Model file for the job. Use its own axes, mm. A direction names the side the tool comes from. Coordinates: 2 decimals unless noted, no trailing zeros. Loops run counter-clockwise (first coordinate to the right, second up) from the corner with the lowest first, then second, coordinate; pieces in that order, holes last.
from build123d import *

# Parameters (mm, degrees)
BASE_FLANGE1_DEPTH         = 3.175
M3_5_CLEARANCE_HOLE1_D     = 3.75
F_5_2_5_2_DIAMETER_HOLE1_D = 5.2
F_3_2_3_2_DIAMETER_HOLE1_D = 3.2
M20_CLEARANCE_HOLE1_D      = 22.86


# Sheet-metal steps are written as plain solids
with BuildPart() as part:
    # Sketch11 → Base-Flange1 (new body)
    with BuildSketch(Plane.XY.offset(3.175)):
        with BuildLine():
            Line((-42, 51), (-42, 19))
            ThreePointArc((-42, 19), (-40.535533906, 15.464466094), (-37, 14))
            Line((-37, 14), (-5, 14))
            ThreePointArc((-5, 14), (-1.464466094, 12.535533906), (0, 9))
            Line((0, 9), (0, 5))
            ThreePointArc((0, 5), (1.464466094, 1.464466094), (5, 0))
            Line((5, 0), (15, 0))
            ThreePointArc((15, 0), (18.535533906, 1.464466094), (20, 5))
            Line((20, 5), (20, 35.499999523))
            Line((20, 35.499999523), (48, 35.499999523))
            ThreePointArc((48, 35.499999523), (51.535533906, 36.964465617), (53, 40.499999523))
            Line((53, 40.499999523), (53, 50))
            ThreePointArc((53, 50), (51.535533906, 53.535533906), (48, 55))
            Line((48, 55), (20, 55))
            Line((20, 55), (20, 75))
            ThreePointArc((20, 75), (18.535533906, 78.535533906), (15, 80))
            Line((15, 80), (5, 80))
            ThreePointArc((5, 80), (1.464466094, 78.535533906), (0, 75))
            Line((0, 75), (0, 61))
            ThreePointArc((0, 61), (-1.464466094, 57.464466094), (-5, 56))
            Line((-5, 56), (-37, 56))
            ThreePointArc((-37, 56), (-40.535533906, 54.535533906), (-42, 51))
        make_face()
    extrude(amount=-BASE_FLANGE1_DEPTH)

    # M3.5 Clearance Hole1 (through all)
    with Locations(Plane.XY.offset(3.175)):
        with Locations((17, 75), (3, 5), (3, 75), (17, 5)):
            Hole(M3_5_CLEARANCE_HOLE1_D / 2)

    # Ø5.2 (5.2) Diameter Hole1 (through all)
    with Locations(Plane.XY.offset(3.175)):
        with Locations((47.5, 45), (27.5, 45)):
            Hole(F_5_2_5_2_DIAMETER_HOLE1_D / 2)

    # Ø3.2 (3.2) Diameter Hole1 (through all)
    with Locations(Plane.XY.offset(3.175)):
        with Locations((-36.490941809, 50.490941809), (-5.509058191, 50.490941809), (-5.509058191, 19.509058191), (-36.490941809, 19.509058191)):
            Hole(F_3_2_3_2_DIAMETER_HOLE1_D / 2)

    # M20 Clearance Hole1 (through all)
    with Locations(Plane.XY.offset(3.175)):
        with Locations((-21, 35)):
            Hole(M20_CLEARANCE_HOLE1_D / 2)


solid = part.part
Q1. Mould opens along Y. For faces 3 (the flat face through (20, 20, 2)), 4 (the flat face through (10, 80, 2)), 5 (the cylindrical face through (28.06, 42.46, 1.57)) say: +Y half, -Y half, draft (parallel to the pull), parting line (faces both ways), or undercut.
Answers:
face 3: draft
face 4: +Y half
face 5: undercut
Q2. Drill centre lines: line 1 (Y direction, x = 17.5, z = 2.05); line 2 (Y direction, x = 4, z = 2.75); line 3 (Y direction, x = -21, z = 1.15). Where is each one in solid material? Low to high.
Answers:
line 1: y = 0.67 to 3.19, 6.81 to 73.19, 76.81 to 79.33
line 2: y = 0.1 to 3.41, 6.59 to 73.41, 76.59 to 79.9
line 3: y = 14 to 23.57, 46.43 to 56
Q3. Slice it at B-B (y = 31). List the corners of the cut face in (x, z) (3 decimals).
Answers:
outline: (-42, 0) - (-31.707, 0) - (-31.707, 3.175) - (-42, 3.175) - close; (-10.293, 0) - (20, 0) - (20, 3.175) - (-10.293, 3.175) - close
Q4. Slice it at C-C (z = 0.8). Count the separate pieces of the cut face and the enclosed holes in it, and give its area (3 significant figures).
Answers:
separate pieces: 1
enclosed holes: 11
area: 3,450 mm2
Q5. Flat gauge pins, fed straight in: P1, Ø1.6, axis at y = 8, z = 2, coming from the -X side; P2, Ø4, axis at x = -5.51, y = 19.51, coming from the -Z side; P3, Ø1.6, axis at x = -14, z = 2, coming from the -Y side; P4, Ø1.5, axis at x = 32.5, z = 2, coming from the +Y side. Where does each tip first touch, or does it go through?
Answers:
P1: stops at x = 0
P2: stops at z = 0
P3: stops at y = 14
P4: stops at y = 55
Q6. Slice it at A-A (x = 27.5). List the corners of the cut face in (y, z) (3 decimals).
Answers:
outline: (35.5, 0) - (42.4, 0) - (42.4, 3.175) - (35.5, 3.175) - close; (47.6, 0) - (55, 0) - (55, 3.175) - (47.6, 3.175) - close
Q7. Which spindle directions (+Z, -Z, +X, -X, +Y, -Y) get a long thin tool onto all of the face, cutting with end or side? Do faces 1 (the cylindrical face through (51.5, 36.93, 1.61)), 2 (the flat face through (-21, 56, 2)). Say none if no direction does.
Answers:
face 1: +Z, -Z, +X, -Y
face 2: +Z, -Z, -X, +Y
Q8. Slice it at D-D (y = 45). List the corners of the cut face in (x, z) (3 decimals), and give its area (3 significant figures).
Answers:
outline: (-42, 0) - (-26.536, 0) - (-26.536, 3.175) - (-42, 3.175) - close; (-15.464, 0) - (24.9, 0) - (24.9, 3.175) - (-15.464, 3.175) - close; (30.1, 0) - (44.9, 0) - (44.9, 3.175) - (30.1, 3.175) - close; (50.1, 0) - (53, 0) - (53, 3.175) - (50.1, 3.175) - close
area: 233 mm2
